from build123d import *

# Parameters (mm, degrees)
SKETCH_R              = 50
PAD_DEPTH             = 3
SKETCH004_R           = 5.2
POCKET001_DEPTH       = 3.001
POCKET002_DEPTH       = 3.001
SKETCH006_R           = 50
SKETCH006_R_2         = 46
PAD001_DEPTH          = 17.5
POCKET003_DEPTH       = 3
POLARPATTERN001_COUNT = 3
PAD002_DEPTH          = 2.8
POLARPATTERN002_COUNT = 3


with BuildPart() as part:
    # Sketch → Pad (new body)
    with BuildSketch(Plane.XY):
        Circle(SKETCH_R)
    extrude(amount=PAD_DEPTH)

    # Sketch004 (on DatumPlane) → Pocket001 (cut, through all)
    with BuildSketch(Plane.XY.offset(3)):
        Circle(SKETCH004_R)
    extrude(amount=-POCKET001_DEPTH, mode=Mode.SUBTRACT)

    # Sketch005 → Pocket002 (cut, through all)
    with BuildSketch(Plane.XY):
        with BuildLine():
            ThreePointArc((33.2768944622, -31.7592237776), (39.8371685741, -23), (44.1427418269, -12.9390240745))
            Line((23.8754986114, -7.4135393744), (44.1427418269, -12.9390240745))
            ThreePointArc((18.3580627359, -16.9700186383), (21.6506350946, -12.5), (23.8754986114, -7.4135393744))
            Line((33.2768944622, -31.7592237776), (18.3580627359, -16.9700186383))
        make_face()
    extrude(amount=POCKET002_DEPTH, mode=Mode.SUBTRACT)

    # Sketch006 → Pad001 (join)
    with BuildSketch(Plane.XY):
        Circle(SKETCH006_R)
        Circle(SKETCH006_R_2, mode=Mode.SUBTRACT)
    extrude(amount=-PAD001_DEPTH)

    # Sketch007 (on DatumPlane) → Pocket003 (cut)
    with BuildSketch(Plane.XY.offset(3)):
        with BuildLine():
            ThreePointArc((45.3011566386, -7.9878161727), (46, 0), (45.3011566386, 7.9878161727))
            Line((45.3011566386, 7.9878161727), (47.2707721446, 8.335112528))
            ThreePointArc((47.2707721446, -8.335112528), (48, 0), (47.2707721446, 8.335112528))
            Line((47.2707721446, -8.335112528), (45.3011566386, -7.9878161727))
        make_face()
    pocket003 = extrude(amount=-POCKET003_DEPTH, mode=Mode.SUBTRACT)

    # PolarPattern001: Pocket003 ×3 about axis
    polarpattern001_axis = Axis((0, 0, 3), (0, 0, 1))
    for i in range(1, POLARPATTERN001_COUNT):
        add(pocket003.rotate(polarpattern001_axis, i * 360 / POLARPATTERN001_COUNT), mode=Mode.SUBTRACT)

    # Sketch008 (on DatumPlane) → Pad002 (join)
    with BuildSketch(Plane.XY.offset(-17.5)):
        with BuildLine():
            ThreePointArc((-45.3691376707, 7.5921898696), (-46, 0), (-45.3691376707, -7.5921898696))
            Line((-47.1444517535, -7.8892755601), (-45.3691376707, -7.5921898696))
            ThreePointArc((-47.1444517535, 7.8892755601), (-47.8, 0), (-47.1444517535, -7.8892755601))
            Line((-45.3691376707, 7.5921898696), (-47.1444517535, 7.8892755601))
        make_face()
    pad002 = extrude(amount=-PAD002_DEPTH)

    # PolarPattern002: Pad002 ×3 about axis
    polarpattern002_axis = Axis((0, 0, -17.5), (0, 0, 1))
    for i in range(1, POLARPATTERN002_COUNT):
        add(pad002.rotate(polarpattern002_axis, i * 360 / POLARPATTERN002_COUNT))


solid = part.part
Geometry check sheet. Reference: the model listing, model coordinates, mm. A direction names the side the tool comes from. Coordinates: 2 decimals unless noted, no trailing zeros. Order: outer loops, then holes, each group sorted by start corner. A loop starts at its lowest first (then second) coordinate and runs counter-clockwise, first axis right, second up. Notation, with made-up numbers: (64.5, -36) -> (119.5, -36) arc R35 cw to (119.5, -3) -> close; hole circle Ø11 at (63, 28.25). An arc over 180 degrees is marked (long way). Use a Markdown table: item, result. Add a question column.
1. Go/stop test with flat-tipped pins: pin 1 Ø2 at (x, z) = (0, -11) entering from -Y; pin 2 Ø8.5 at (x, y) = (0, 0) entering from -Z; pin 3 Ø10 at (y, z) = (39.5, -17) entering from +X; pin 4 Ø1.5 at (y, z) = (-12, -16) entering from +X. Record where each tip stops, or that it passes through.
2. Material ranges on L1, parallel to Y at x = 0, z = 1.8; L2, parallel to Y at x = 0, z = -14; L3, parallel to Z at x = -28, y = 3, recorded low to high.
3. Mould release check, pull along Y, two halves, no side actions. Record for faces 1 (the face through (48, 0, 2)), 2 (the face through (24, 41.34, -18.88)), 3 (the face through (23.2, -40.4, -20.3)): pulls with the +Y half, pulls with the -Y half, needs draft (parallel to the pull), parting line crosses it, or undercut.
4. Cross-section at D-D (y = 30). Enter the section's corners in (x, z), and give its area (3 significant figures).
5. Cross-section at B-B (x = 0). Enter the section's corners in (y, z), and give its area (3 significant figures).
6. Cross-section at C-C (z = -5). Enter the section's corners in (x, y).
7. Set-up check for faces 4 (the face through (-1, -10, 0)), 5 (the face through (33.87, -10.14, 1.48)), 6 (the face through (-23.4, 40.4, 0)), 7 (the face through (-47.8, 0.1, -18.9)), 8 (the face through (23.804, -41.451, -18.88)): record each of +Z, -Z, +X, -X, +Y, -Y from which the full face is reachable in a straight line by a thin tool's end or side.
Filled sheet:
| question | item | result |
|---|---|---|
| 1 | pin 1 | y = -50 |
| 1 | pin 2 | through |
| 1 | pin 3 | x = 36.19 |
| 1 | pin 4 | x = 48.72 |
| 2 | L1 | -50 to -5.2, 5.2 to 50 |
| 2 | L2 | -50 to -46, 46 to 50 |
| 2 | L3 | 0 to 3 |
| 3 | face 1 | undercut |
| 3 | face 2 | pulls with the +Y half |
| 3 | face 3 | needs draft |
| 4 | outline | (-40, -17.5) -> (-34.87, -17.5) -> (-34.87, 0) -> (34.87, 0) -> (34.87, -17.5) -> (40, -17.5) -> (40, 3) -> (-40, 3) -> close |
| 4 | area | 420 mm2 |
| 5 | outline | (-50, -17.5) -> (-46, -17.5) -> (-46, 0) -> (-5.2, 0) -> (-5.2, 3) -> (-50, 3) -> close; (5.2, 0) -> (46, 0) -> (46, -17.5) -> (50, -17.5) -> (50, 3) -> (5.2, 3) -> close |
| 5 | area | 409 mm2 |
| 6 | outline | circle Ø100 at (0, 0); hole circle Ø92 at (0, 0) |
| 7 | face 4 | -Z |
| 7 | face 5 | +Z, -Z |
| 7 | face 6 | +Z |
| 7 | face 7 | -Z, -X |
| 7 | face 8 | -Z, +X, -Y |
